Autodesk Inventor part; units mm, degrees
ref_plane "YZ Plane" through (0, 0, 0) normal (1, 0, 0) x (0, 1, 0)
ref_plane "XZ Plane" through (0, 0, 0) normal (0, 1, 0) x (-1, 0, 0)
ref_plane "XY Plane" through (0, 0, 0) normal (0, 0, 1) x (1, 0, 0)
sketch "Sketch1" plane through (0, 0, 0) normal (0, 1, 0) x (-1, 0, 0)
  line L0 (-11, -15) -> (-11, 15)
  line L1 (-11, 15) -> (11, 15)
  arc A0 (-11, -15) -> (11, 15) centre (-20.4545, 15) ccw
  line L2 (11, 15) -> (-11, 15)
  line L3 (-11, 15) -> (-11, 40)
  line L4 (-11, 40) -> (11, 40)
  line L5 (11, 40) -> (11, 15)
  line L6 (11, 40) -> (-11, 40)
  line L7 (-11, 40) -> (-11, 55)
  line L8 (-11, 55) -> (11, 55)
  line L9 (11, 55) -> (11, 40)
  circle A1 centre (0, 47.5) radius 0.1
  line L10 (-11, 15) -> (-3, 15)
  circle A2 centre (-3, 7) radius 0.1
  circle A3 centre (-3, -1) radius 0.1
  dimension "d0" = 22
  dimension "d1" = 30
  dimension "d2" = 25
  dimension "d3" = 15
  dimension "d4" = 0.2
  dimension "d5" = 8
  dimension "d8" = 0.2
  dimension "d10" = 0.2
extrude "Extrusion1" add sketch "Sketch1" along normal blind 2
properties part number "drzak_buzirka1"
Here's how the part is built. I have some questions about the finished solid (model axes, mm). Coordinates: 2 decimals unless noted, no trailing zeros. Order: outer loops, then holes, each group sorted by start corner. A loop starts at its lowest first (then second) coordinate and runs counter-clockwise, first axis right, second up. Notation, with made-up numbers: (-38, -21) -> (-19, -21) arc R8 ccw to (-19, -14) -> close; hole circle Ø6 at (8, -16.5). An arc over 180 degrees is marked (long way). Answer in a Markdown table with one row per item.
(1) I want a section at B-B on x = -1. List the corners of the cut face in (y, z) for me, then the cut area to 3 significant figures.
Answer key:
| item | result |
|---|---|
| outline | (0, -8) -> (2, -8) -> (2, 55) -> (0, 55) -> close |
| area | 126 mm^2 |
(2) I want a section at A-A on y = 1.4. List the corners of the cut face in (x, z) for me, then the cut area to 3 significant figures.
Answer key:
| item | result |
|---|---|
| outline | (-11, 15) arc R31.45 ccw to (11, -15) -> (11, 55) -> (-11, 55) -> close; hole circle Ø0.2 at (0, 47.5); hole circle Ø0.2 at (3, -1); hole circle Ø0.2 at (3, 7) |
| area | 1,360 mm^2 |
(3) I want a section at C-C on x = -5.5. List the corners of the cut face in (y, z) for me.
Answer key:
| item | result |
|---|---|
| outline | (0, -2.77) -> (2, -2.77) -> (2, 55) -> (0, 55) -> close |
(4) Will this pin go through, and if not, where does the flat tip stop? pin 1 Ø8 at (x, z) = (-6, 14) entering from -Y.
Answer key:
| item | result |
|---|---|
| pin 1 | y = 0 |
(5) Please list where these lines run through material, in increasing order: probe 1 along X at (y, z) = (0.85, 47.5); probe 2 along Z at (x, y) = (3, 1.5); probe 3 along Z at (x, y) = (0, 1.5).
Answer key:
| item | result |
|---|---|
| probe 1 | -11 to -0.1, 0.1 to 11 |
| probe 2 | -11.17 to -1.1, -0.9 to 6.9, 7.1 to 55 |
| probe 3 | -8.9 to 47.4, 47.6 to 55 |
